```python
from build123d import *

# Parameters (mm, degrees)
ESQUISSE1_R             = 3.5
ESQUISSE1_R_2           = 1.5
BOSS_EXTRU_1_DEPTH      = 5
CONG_1_R                = 0.2
ESQUISSE3_R             = 3.3
ESQUISSE3_R_2           = 1.7
ENL_V_MAT_EXTRU_1_DEPTH = 0.5
ESQUISSE4_R             = 3.3
ESQUISSE4_R_2           = 1.7
ENL_V_MAT_EXTRU_2_DEPTH = 0.5


with BuildPart() as part:
    # Esquisse1 → Boss.-Extru.1 (new body)
    with BuildSketch(Plane(origin=(0, 0, 0), x_dir=(1, 0, 0), z_dir=(0, 1, 0))):
        Circle(ESQUISSE1_R)
        Circle(ESQUISSE1_R_2, mode=Mode.SUBTRACT)
    extrude(amount=BOSS_EXTRU_1_DEPTH)

    # Congé1
    cong_1_edges = [part.edges().sort_by_distance(p)[0] for p in [
        (-3.5, 0, 0),
        (-3.5, 5, 0),
        (-1.5, 0, 0),
        (-1.5, 5, 0),
    ]]
    fillet(cong_1_edges, radius=CONG_1_R)

    # Esquisse3 → Enlèv. mat.-Extru.1 (cut)
    with BuildSketch(Plane(origin=(0, 5, 0), x_dir=(1, 0, 0), z_dir=(0, 1, 0))):
        Circle(ESQUISSE3_R)
        Circle(ESQUISSE3_R_2, mode=Mode.SUBTRACT)
    extrude(amount=-ENL_V_MAT_EXTRU_1_DEPTH, mode=Mode.SUBTRACT)

    # Esquisse4 → Enlèv. mat.-Extru.2 (cut)
    with BuildSketch(Plane.XZ):
        Circle(ESQUISSE4_R)
        Circle(ESQUISSE4_R_2, mode=Mode.SUBTRACT)
    extrude(amount=-ENL_V_MAT_EXTRU_2_DEPTH, mode=Mode.SUBTRACT)


solid = part.part
```
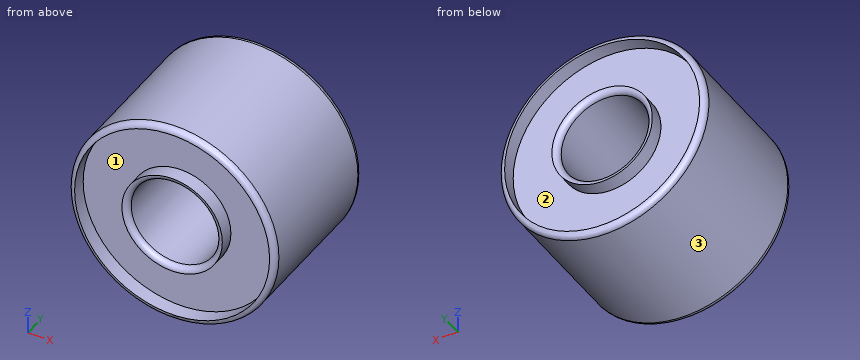
Part model, mm, in its own coordinate system. Face numbers are marked on the shaded views. Coordinates: 2 decimals unless noted, no trailing zeros. Order: outer loops, then holes, each group sorted by start corner. A loop starts at its lowest first (then second) coordinate and runs counter-clockwise, first axis right, second up. Notation, with made-up numbers: (43, 24) - (70, 24) arc R20 cw to (70, 46) - close; hole circle Ø8 at (-37.75, 43). An arc over 180 degrees is marked (long way). Return JSON: item names as keys, results as strings. Group by question number.
Item 1: Cut at A-A (x = 0). List the corners of the cut face in (y, z).
Item 2: Cut at C-C (y = 1.8). List the corners of the cut face in (x, z).
Item 3: Drill centre lines: probe 1 along X at (y, z) = (0.3, 0); probe 2 along X at (y, z) = (1.1, 0). Where is each one in solid material? Low to high. Write a range as from..to.
Item 4: Pin check, flat tip, straight feed: pin 1 (1.5 mm diameter, centred on x = -2, z = 1.5, fed in from +Y). Stop position of the tip, or through.
Item 5: Cut at B-B (z = 0). List the corners of the cut face in (x, y).
Item 6: Pull direction Z, two halves, no side cores. Call the marked faces 1, 2 and 3: pulls with the +Z half, pulls with the -Z half, needs draft (parallel to the pull), parting line crosses it, or undercut.
Check values:
{
 "1": {"outline": "(0, -3.3) arc R0.2 ccw to (0.2, -3.5) - (4.8, -3.5) arc R0.2 ccw to (5, -3.3) - (4.5, -3.3) - (4.5, -1.7) - (5, -1.7) arc R0.2 ccw to (4.8, -1.5) - (0.2, -1.5) arc R0.2 ccw to (0, -1.7) - (0.5, -1.7) - (0.5, -3.3) - close; (0, 1.7) arc R0.2 ccw to (0.2, 1.5) - (4.8, 1.5) arc R0.2 ccw to (5, 1.7) - (4.5, 1.7) - (4.5, 3.3) - (5, 3.3) arc R0.2 ccw to (4.8, 3.5) - (0.2, 3.5) arc R0.2 ccw to (0, 3.3) - (0.5, 3.3) - (0.5, 1.7) - close"},
 "2": {"outline": "circle Ø7 at (0, 0); hole circle Ø3 at (0, 0)"},
 "3": {"probe 1": "x = -3.5..-3.3, -1.7..-1.5, 1.5..1.7, 3.3..3.5", "probe 2": "x = -3.5..-1.5, 1.5..3.5"},
 "4": {"pin 1": "stops at y = 4.5"},
 "5": {"outline": "(-3.5, 0.2) arc R0.2 ccw to (-3.3, 0) - (-3.3, 0.5) - (-1.7, 0.5) - (-1.7, 0) arc R0.2 ccw to (-1.5, 0.2) - (-1.5, 4.8) arc R0.2 ccw to (-1.7, 5) - (-1.7, 4.5) - (-3.3, 4.5) - (-3.3, 5) arc R0.2 ccw to (-3.5, 4.8) - close; (1.5, 0.2) arc R0.2 ccw to (1.7, 0) - (1.7, 0.5) - (3.3, 0.5) - (3.3, 0) arc R0.2 ccw to (3.5, 0.2) - (3.5, 4.8) arc R0.2 ccw to (3.3, 5) - (3.3, 4.5) - (1.7, 4.5) - (1.7, 5) arc R0.2 ccw to (1.5, 4.8) - close"},
 "6": {"face 1": "undercut", "face 2": "undercut", "face 3": "parting line crosses it"}
}
